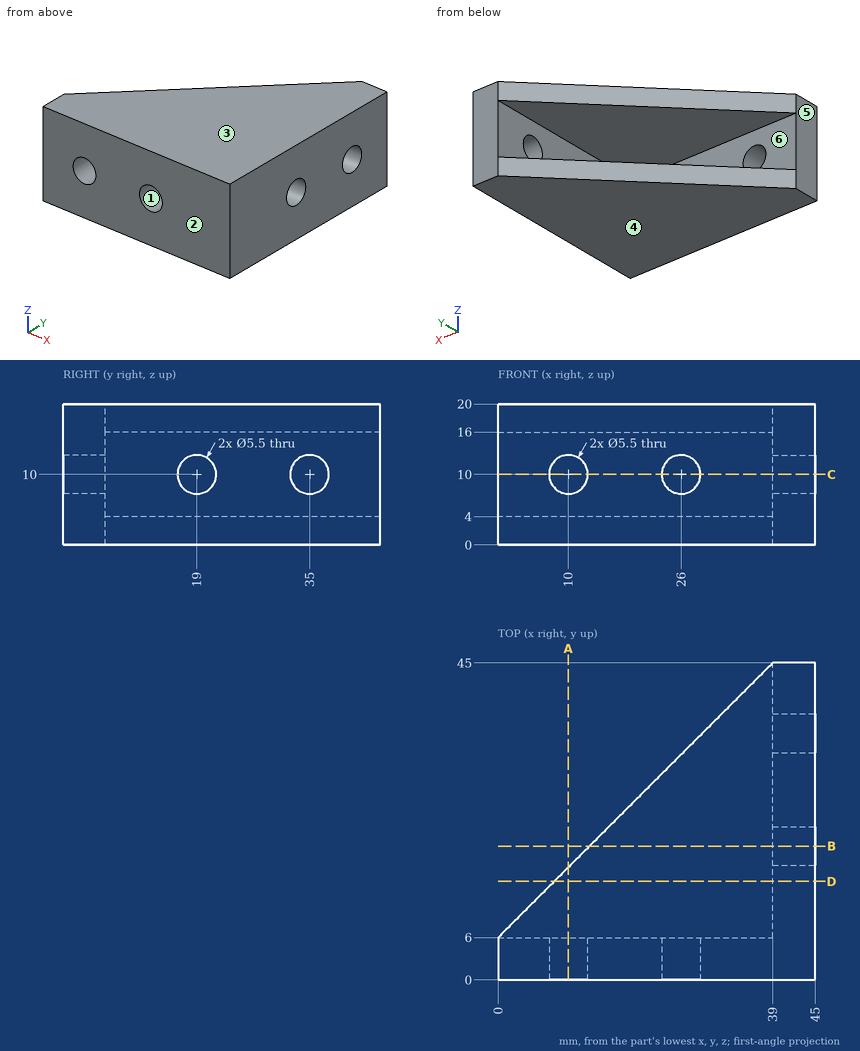
Verification items for this drawing (mm, ordinates from the low corner). A direction names the side the tool comes from. Give positions to 0.01 mm unless a question says otherwise; leave off trailing zeros. Loops run counter-clockwise (first coordinate to the right, second up) from the corner with the lowest first, then second, coordinate; pieces in that order, holes last. Notation, with made-up numbers: (-27.5, -22) - (11.5, -22) arc R9 cw to (11.5, -17) - close; hole circle Ø10 at (48, 25.25). An arc over 180 degrees is marked (long way). Write item = value, one per line. Start each with the question number.
Q1. Cross-section at D-D, the plane y = 14. Enter the section's corners in (x, z), and give its area (3 significant figures).
Q2. Depth check by flat-ended pin: P1, Ø12, axis at y = 26.5, z = 13.5, coming from the -X side; P2, Ø8, axis at x = 38, z = 2.5, coming from the +Y side; P3, Ø12, axis at y = 19, z = 8.5, coming from the -X side; P4, Ø6, axis at x = 28.5, z = 9, coming from the +Y side. Enter the tip coordinate at first touch or a pass-through.
Q3. Cross-section at B-B, the plane y = 19. Enter the section's corners in (x, z).
Q4. Cross-section at A-A, the plane x = 10. Enter the section's corners in (y, z), and give its area (3 significant figures).
Q5. Cross-section at C-C, the plane z = 10. Enter the section's corners in (x, y).
Q6. Thickness scan on line 1 (Y direction, x = 43.2, z = 10); line 2 (Z direction, x = 10, y = 2.2); line 3 (Y direction, x = 43.5, z = 12.5). Record the ranges inside material, lowest first.
Q7. Tool access check on the marked faces 5 and 6. Record the directions out of +Z, -Z, +X, -X, +Y, -Y that give a thin tool (end or side, any length) a straight path to the whole face; none if there is none.
Q8. Mould release check, pull along Z, two halves, no side actions. Record for the marked faces 1, 2, 3 and 4: released by +Z, released by -Z, zero draft, split by the parting line, or undercut.
Answer key:
q1.outline = (8, 0) - (45, 0) - (45, 20) - (8, 20) - (8, 16) - (39, 16) - (39, 4) - (8, 4) - close
q1.area = 368 mm^2
q2.P1 = 15.05
q2.P2 = 45
q2.P3 = 9.03
q2.P4 = 6
q3.outline = (13, 0) - (45, 0) - (45, 7.25) - (39, 7.25) - (39, 4) - (13, 4) - close; (13, 16) - (39, 16) - (39, 12.75) - (45, 12.75) - (45, 20) - (13, 20) - close
q4.outline = (0, 0) - (16, 0) - (16, 4) - (6, 4) - (6, 7.25) - (0, 7.25) - close; (0, 12.75) - (6, 12.75) - (6, 16) - (16, 16) - (16, 20) - (0, 20) - close
q4.area = 167 mm^2
q5.outline = (0, 0) - (7.25, 0) - (7.25, 6) - (0, 6) - close; (12.75, 0) - (23.25, 0) - (23.25, 6) - (12.75, 6) - close; (28.75, 0) - (45, 0) - (45, 16.25) - (39, 16.25) - (39, 6) - (28.75, 6) - close; (39, 21.75) - (45, 21.75) - (45, 32.25) - (39, 32.25) - close; (39, 37.75) - (45, 37.75) - (45, 45) - (39, 45) - close
q6.line_1 = 0 to 16.25, 21.75 to 32.25, 37.75 to 45
q6.line_2 = 0 to 7.25, 12.75 to 20
q6.line_3 = 0 to 17.85, 20.15 to 33.85, 36.15 to 45
q7.face_5 = +Z, -Z, -X, +Y, -Y
q7.face_6 = -X, +Y
q8.face_1 = undercut
q8.face_2 = zero draft
q8.face_3 = released by +Z
q8.face_4 = released by -Z
